from build123d import *

# Parameters (mm, degrees)
F0_W        = 46.0375
F0_H        = 44.45
F1_DEPTH    = 7.9375
F2_T1_DEPTH = 87.1311818198
F3_T        = -1.905
F5_D        = 4.445


# Not quite as in the source:
# - a fillet or chamfer that OpenCascade refuses, or shapes differently, is made with other operations: its cross-section is extruded or revolved along the edge and cut away or added


with BuildPart() as f1:
    # F0 (on Top) → F1 (new body)
    with BuildSketch(Plane.XY):
        with Locations((3.8099996746, 17.1172746531)):
            Rectangle(F0_W, F0_H)
    extrude(amount=F1_DEPTH)

    # F2: chamfer of 4.7625 x 8.248891971 on 2 edges, made by hand

    # F2_s2 → F2_t1 (cut)
    with BuildSketch(Plane.XZ.offset(-60.682865563)):
        Polygon((-19.2087503254, -0.311391971), (-14.4462503254, 7.9375), (-19.2087503254, 7.9375), align=None)
        Polygon((26.8287496746, -0.311391971), (22.0662496746, 7.9375), (26.8287496746, 7.9375), align=None)
    extrude(amount=F2_T1_DEPTH, mode=Mode.SUBTRACT)

    # F3
    f3_openings = [f1.faces().sort_by_distance(p)[0] for p in [
        (3.81, 17.117275, 0),
    ]]
    offset(amount=F3_T, openings=f3_openings)

    # F5 (through all)
    with Locations(Plane.XY.offset(7.9375)):
        with Locations((3.8099996746, 17.1172746531)):
            Hole(F5_D / 2)


solid = f1.part
Can you work these out from the model? Positions are in its coordinate system, mm. A direction names the side the tool comes from. Round coordinates to 2 decimals unless told otherwise and drop trailing zeros. Write each loop counter-clockwise with the first axis right and the second up, starting at its lowest first coordinate (ties: lowest second). Pieces come first, ordered by that corner, then holes. Notation, with made-up numbers: M 33,10 L 76,10 A14 ccw 76,15 Z; hole C 68.5,49 d3. An arc over 180 degrees is marked long. Use CSV: the item, a comma, the result in double quotes.
(1) Imagine slicing it at A-A (x = 3.81). Write out the boundary of the cut face in (y, z).
Check values:
outline,"M -5.11,0 L -3.2,0 L -3.2,6.03 L 14.89,6.03 L 14.89,7.94 L -5.11,7.94 Z; M 19.34,6.03 L 37.44,6.03 L 37.44,0 L 39.34,0 L 39.34,7.94 L 19.34,7.94 Z"
(2) I'm going to push flat-ended pins straight in: pin 1 (2 mm diameter, centred on y = 30, z = 5, fed in from -X); pin 2 (1 mm diameter, centred on y = 15, z = 1.5, fed in from +X); pin 3 (17 mm diameter, centred on x = -4.5, y = 21.5, fed in from -Z). Where does each tip first touch, or does it pass through?
Check values:
pin 1,"x = -16.72"
pin 2,"x = 26.07"
pin 3,"z = 6.03"
(3) Imagine slicing it at B-B (z = 3). Write out the boundary of the cut face in (x, y), plus the area to 3 significant figures.
Check values:
outline,"M -17.3,-5.11 L 24.92,-5.11 L 24.92,39.34 L -17.3,39.34 Z; hole M -15.1,-3.2 L 22.72,-3.2 L 22.72,37.44 L -15.1,37.44 Z"
area,"340 mm^2"
(4) Imagine slicing it at C-C (y = 35.5). Write out the boundary of the cut face in (x, z), plus the area to 3 significant figures.
Check values:
outline,"M -19.03,0 L -16.83,0 L -13.35,6.03 L 20.97,6.03 L 24.45,0 L 26.65,0 L 22.07,7.94 L -14.45,7.94 Z"
area,"98.2 mm^2"
(5) I need wall thicknesses on line 1 along Y through (x, z) = (-9.5, 4); line 2 along Y through (x, z) = (3.81, 7.2); line 3 along X through (y, z) = (23, 2.25). Which ranges of each line are inside material? Lowest first, please.
Check values:
line 1,"-5.11 to -3.2, 37.44 to 39.34"
line 2,"-5.11 to 14.89, 19.34 to 39.34"
line 3,"-17.73 to -15.53, 23.15 to 25.35"
(6) We'd pull the mould along X, two halves only. Please class faces 1 (the flat face through (22.732, 17.402, 2.974)), 2 (the flat face through (24.39, 17.43, 3.91)), 3 (the flat face through (3, 39.342, 4)), 4 (the flat face through (-16.77, 17.43, 3.91)): +X half, -X half, draft (parallel to the pull), parting line (faces both ways), or undercut.
Check values:
face 1,"undercut"
face 2,"+X half"
face 3,"draft"
face 4,"-X half"
(7) Imagine slicing it at D-D (x = 15). Write out the boundary of the cut face in (y, z), plus the area to 3 significant figures.
Check values:
outline,"M -5.11,0 L -3.2,0 L -3.2,6.03 L 37.44,6.03 L 37.44,0 L 39.34,0 L 39.34,7.94 L -5.11,7.94 Z"
area,"108 mm^2"
(8) On a 3-axis mill with a long thin cutter (end or side, diameter ignored), from which of +Z, -Z, +X, -X, +Y, -Y can I reach the whole of each face in a straight line? I mean faces 5 (the flat face through (2, -4, 0)), 6 (the flat face through (4, -3.203, 3)). Say none if no direction works.
Check values:
face 5,"-Z, +X, -X, +Y, -Y"
face 6,"-Z"
